Could you check a few things on this model? Use its own coordinates, in mm. Face numbers are marked on the shaded views. A direction names the side the tool comes from. Give positions to 0.01 mm unless a question says otherwise; leave off trailing zeros. Order: outer loops, then holes, each group sorted by start corner. A loop starts at its lowest first (then second) coordinate and runs counter-clockwise, first axis right, second up. Notation, with made-up numbers: M -39,25.5 L 11,25.5 A26 cw 11,64.5 Z; hole C 37,76.25 d4. An arc over 180 degrees is marked long. Return JSON: item names as keys, results as strings. Group by question number.
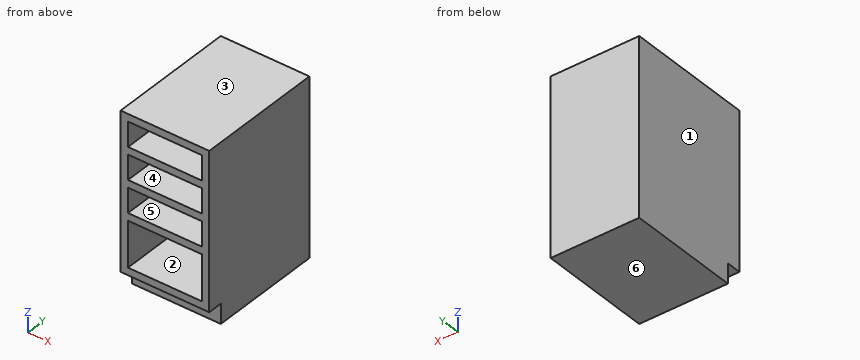
```python
from build123d import *

# Parameters (mm, degrees)
F1_DEPTH = 457.2
F2_W     = 381
F2_H     = 127
F2_H_2   = 234.95
F3_DEPTH = 596.9


with BuildPart() as f1:
    # F0 (on Right) → F1 (new body)
    with BuildSketch(Plane.YZ):
        Polygon((-584.2, 0), (0, 0), (0, 908.05), (-660.4, 908.05), (-660.4, 101.6), (-584.2, 101.6), align=None)
    extrude(amount=F1_DEPTH)

    # F2 (on face) → F3 (cut)
    with BuildSketch(Plane.XZ.offset(660.4)):
        with Locations((228.6, 806.45)):
            Rectangle(F2_W, F2_H)
        with Locations((228.6, 641.35)):
            Rectangle(F2_W, F2_H)
        with Locations((228.6, 476.25)):
            Rectangle(F2_W, F2_H)
        with Locations((228.6, 257.175)):
            Rectangle(F2_W, F2_H_2)
    extrude(amount=-F3_DEPTH, mode=Mode.SUBTRACT)


solid = f1.part
```
1. Imagine slicing it at C-C, the plane x = 83. Please give me the cut outline in (y, z), plus the area to 3 significant figures.
2. Imagine slicing it at A-A, the plane y = -397. Please give me the cut outline in (x, z).
3. I need wall thicknesses on L1, parallel to Z at x = 327.5, y = -421; L2, parallel to Z at x = 161.5, y = -605; L3, parallel to X at y = -277, z = 520. Which ranges of each line are inside material? Lowest first, please. Write a range as from..to.
4. Which directions (+Z, -Z, +X, -X, +Y, -Y) give clear straight access to the entire face, cutting with the end or side of a thin tool? Please do the marked faces 5 and 6.
5. For pin 1 (3 mm diameter, centred on x = 339.5, z = 255, fed in from -Y), with a flat end and sliding along its axis, tell me the tip position at first contact or that it passes through.
6. If we mould it in two halves opening along X, with no side actions, what happens to the marked faces 1, 2, 3 and 4? For each: pulls with the +X half, pulls with the -X half, needs draft (parallel to the pull), parting line crosses it, or undercut.
7. Imagine slicing it at B-B, the plane z = 595.5. Please give me the cut outline in (x, y), plus the area to 3 significant figures.
8. Imagine slicing it at D-D, the plane z = 91. Please give me the cut outline in (x, y), plus the area to 3 significant figures.
Values:
{
 "1": {"outline": "M -660.4,101.6 L -584.2,101.6 L -584.2,0 L 0,0 L 0,908.05 L -660.4,908.05 L -660.4,869.95 L -63.5,869.95 L -63.5,742.95 L -660.4,742.95 L -660.4,704.85 L -63.5,704.85 L -63.5,577.85 L -660.4,577.85 L -660.4,539.75 L -63.5,539.75 L -63.5,412.75 L -660.4,412.75 L -660.4,374.65 L -63.5,374.65 L -63.5,139.7 L -660.4,139.7 Z", "area": "224,000 mm²"},
 "2": {"outline": "M 0,0 L 457.2,0 L 457.2,908.05 L 0,908.05 Z; hole M 38.1,139.7 L 419.1,139.7 L 419.1,374.65 L 38.1,374.65 Z; hole M 38.1,412.75 L 419.1,412.75 L 419.1,539.75 L 38.1,539.75 Z; hole M 38.1,577.85 L 419.1,577.85 L 419.1,704.85 L 38.1,704.85 Z; hole M 38.1,742.95 L 419.1,742.95 L 419.1,869.95 L 38.1,869.95 Z"},
 "3": {"L1": "z = 0..139.7, 374.65..412.75, 539.75..577.85, 704.85..742.95, 869.95..908.05", "L2": "z = 101.6..139.7, 374.65..412.75, 539.75..577.85, 704.85..742.95, 869.95..908.05", "L3": "x = 0..38.1, 419.1..457.2"},
 "4": {"face 5": "-Y", "face 6": "-Z, +X, -X, +Y, -Y"},
 "5": {"pin 1": "stops at y = -63.5"},
 "6": {"face 1": "pulls with the -X half", "face 2": "undercut", "face 3": "needs draft", "face 4": "undercut"},
 "7": {"outline": "M 0,-660.4 L 38.1,-660.4 L 38.1,-63.5 L 419.1,-63.5 L 419.1,-660.4 L 457.2,-660.4 L 457.2,0 L 0,0 Z", "area": "74,500 mm²"},
 "8": {"outline": "M 0,-584.2 L 457.2,-584.2 L 457.2,0 L 0,0 Z", "area": "267,000 mm²"}
}
